Autodesk Fusion 360 part; units mm, degrees
sketch "Sketch1" plane through (0, 0, 0) normal (0, 0, 1) x (1, 0, 0) in component "test"
  line L0 (-10, 10) -> (5, 10)
  line L1 (5, 10) -> (5, 0)
  line L2 (5, 0) -> (-10, 0)
  line L3 (-10, 0) -> (-10, 10)
  line L4 (5, 0) -> (10, 0)
  line L5 (10, 0) -> (5, 2.5)
  dimension "d1" = 15
  dimension "d2" = 10
extrude "Extrude1" add sketch "Sketch1" along normal blind 0.5 in component "test"
sketch "Sketch2" plane through (0, 0, 0.5) normal (0, 0, 1) x (-1, 0, 0) in component "test"
  line L0 (10, 0) -> (-10, 0)
  line L1 (-5, -2.5) -> (-5, -10)
  line L2 (-5, -10) -> (10, -10)
  line L3 (10, -10) -> (10, 0)
  line L4 (10, -10) -> (9, -10)
  line L5 (9, -10) -> (9, 0)
  line L6 (9, 0) -> (10, 0)
  line L7 (10, 0) -> (10, -10)
  line L8 (-5, -10) -> (5, -10)
  line L9 (5, -10) -> (5, -8)
  line L10 (5, -8) -> (-5, -8)
  line L11 (-5, -8) -> (-5, -10)
  line L12 (-10, 0) -> (-5, -2.5)
extrude "Extrude2" add sketch "Sketch2" along normal blind 2 contours L0 L2 L3 L4 L5 L6 L7 | L1 L2 L8 L9 L10 L11 in component "test"
sketch "Sketch3" plane through (0, 0, 2.5) normal (0, 0, 1) x (-1, 0, 0) in component "test"
  line L0 (-5, -8) -> (-5, -10)
  line L1 (-5, -10) -> (5, -10)
  line L2 (5, -10) -> (5, -8)
  line L3 (5, -8) -> (-5, -8)
  line L4 (-5, -8) -> (4, -8)
  line L5 (4, -8) -> (4, -9)
  line L6 (4, -9) -> (-5, -9)
  line L7 (-5, -9) -> (-5, -8)
extrude "Extrude3" cut sketch "Sketch3" against normal blind 1.5 contours L0 L3 L4 L5 L6 L7 in component "test"
sketch "Sketch4" plane through (0, 0, 0.5) normal (0, 0, 1) x (-1, 0, 0) in component "test"
  line L0 (5, -8) -> (5, -10)
  line L1 (5, -10) -> (9, -10)
  line L2 (9, -10) -> (9, 0)
  line L3 (9, 0) -> (-10, 0)
  line L4 (-5, -2.5) -> (-5, -8)
  line L5 (-5, -8) -> (5, -8)
  line L6 (0, -7) -> (4, -7)
  line L7 (4, -7) -> (4, -2)
  line L8 (4, -2) -> (0, -2)
  line L9 (0, -2) -> (0, -7)
  circle A0 centre (6.5, -6.5) radius 1.5
  circle A1 centre (6.5, -2.5) radius 1
  line L10 (-10, 0) -> (-5, -2.5)
  dimension "d9" = 3
  dimension "d10" = 2
extrude "Extrude4" cut sketch "Sketch4" against normal through all contours L6 L7 L8 L9 | A0 | A1 in component "test"
sketch "Sketch5" plane through (0, 0, 2.5) normal (0, 0, 1) x (-1, 0, 0) in component "test"
  line L0 (10, 0) -> (9, 0)
  line L1 (9, 0) -> (9, -10)
  line L2 (9, -10) -> (10, -10)
  line L3 (10, -10) -> (10, 0)
  line L4 (10, -10) -> (2.5, -10)
  line L5 (2.5, -10) -> (2.5, -9)
  line L6 (2.5, -9) -> (10, -9)
  line L7 (10, -9) -> (10, -10)
extrude "Extrude5" add sketch "Sketch5" along normal blind 1 contours L1 L2 L3 L4 L6 L7 | L1 L4 L5 L6 in component "test"
chamfer "Chamfer1" distance 2.5 angle 45 1 edges at (-9.5, 0, 2.5) in component "test"
fillet "Fillet1" radius 2 1 edges at (5, 10, 1.25) in component "test"
fillet "Fillet2" radius 2 1 edges at (-4, 7, 0.25) in component "test"
sketch "Sketch6" plane through (0, 0, 0.5) normal (0, 0, 1) x (-1, 0, 0) in component "test"
  line L0 (9, -0.5) -> (-9, -0.5)
  line L1 (-9, -0.5) -> (-5, -2.5)
  line L2 (-5, -2.5) -> (-5, -8)
  line L3 (-5, -8) -> (5, -8)
  line L4 (5, -8) -> (5, -10)
  line L5 (5, -10) -> (9, -10)
  line L6 (9, -10) -> (9, -0.5)
  line L7 (0, -2) -> (4, -2)
  line L8 (4, -2) -> (4, -5)
  arc A0 (2, -7) -> (4, -5) centre (2, -5) ccw
  line L9 (2, -7) -> (0, -7)
  line L10 (0, -7) -> (0, -2)
  circle A1 centre (6.5, -6.5) radius 1.5
  circle A2 centre (6.5, -2.5) radius 1
  line L11 (5, -8.5) -> (9, -8.5)
  line L12 (9, -8.5) -> (9, -10)
  line L13 (9, -10) -> (5, -10)
  line L14 (5, -10) -> (5, -8.5)
extrude "Extrude6" cut sketch "Sketch6" against normal blind 0.3 contours L4 L5 L6 L11 L12 L13 L14 in component "test"
component "test" placed x (1, 0, 0) y (0, 1, 0) z (0, 0, 1) at (0, 0, 0)
Geometry: final body of the model. Coordinates: model frame, mm. A direction names the side the tool comes from. Round coordinates to 2 decimals unless told otherwise and drop trailing zeros. Order: outer loops, then holes, each group sorted by start corner. A loop starts at its lowest first (then second) coordinate and runs counter-clockwise, first axis right, second up.
Q1. Section C-C, the plane z = 2. Output: boundary loops of the cut face in (x, y).
Result sheet:
outline: (-10, 2) - (-9, 2) - (-9, 10) - (-10, 10) - close; (-5, 8) - (-4, 8) - (-4, 9) - (4.73, 9) arc R2 ccw to (3, 10) - (-5, 10) - close
Q2. Material intervals for probe 1 along Y at (x, z) = (-6.5, 0.25); probe 2 along Y at (x, z) = (-6.5, 0.35); probe 3 along Z at (x, y) = (0.75, 2.5), sorted ascending.
Result sheet:
probe 1: y = 0.25 to 1.5, 3.5 to 5, 8 to 8.5
probe 2: y = 0.35 to 1.5, 3.5 to 5, 8 to 8.5
probe 3: z = 0 to 0.5
Q3. Pin query (flat end, axial travel): pin 1 (0.6 mm diameter, centred on y = 6.5, z = 0, fed in from +X); pin 2 (0.5 mm diameter, centred on y = 8.5, z = 2, fed in from +X); pin 3 (1 mm diameter, centred on x = -3, y = 4, fed in from -Z); pin 4 (0.8 mm diameter, centred on x = 1, y = 9.5, fed in from +Z). Return the tip coordinate at first contact, or that it passes through.
Result sheet:
pin 1: stops at x = 5
pin 2: stops at x = -4
pin 3: passes through
pin 4: stops at z = 2.5
Q4. Access query for faces 1 (the face through (-7, 9.5, 2.5)), 2 (the face through (-4.5, 8.5, 2.5)), 3 (the face through (-2.5, 9.5, 3)), 4 (the face through (0.6, 8.5, 1)). Directions: +Z, -Z, +X, -X, +Y, -Y. A direction counts if a zero-diameter tool reaches every point of the face in a straight line with its end or side. Return the directions, or none.
Result sheet:
face 1: +Y, -Y
face 2: +Z, +X, -X, -Y
face 3: +Z, +X, +Y, -Y
face 4: +Z, +X, -Y
Q5. Section D-D, the plane y = 6.5. Output: boundary loops of the cut face in (x, z), and give its area (3 significant figures).
Result sheet:
outline: (-10, 0) - (-8, 0) - (-8, 0.5) - (-9, 0.5) - (-9, 2.5) - (-10, 2.5) - close; (-5, 0) - (-3.32, 0) - (-3.32, 0.5) - (-5, 0.5) - close; (0, 0) - (5, 0) - (5, 0.5) - (0, 0.5) - close
area: 6.34 mm2
Q6. Mould query, pull axis Y, two halves, no side actions, for faces 5 (the face through (-5.3, 7.4, 0.3)), 6 (the face through (-5.7, 3.1, 0.3)), 7 (the face through (-1.5, 0.3, 0.3)), 8 (the face through (-9.5, 5.7, 2.5)). Classes: released by +Y, released by -Y, zero draft, split by the parting line, or undercut.
Result sheet:
face 5: undercut
face 6: undercut
face 7: released by -Y
face 8: zero draft
Q7. Section B-B, the plane y = 3.75. Output: boundary loops of the cut face in (x, z).
Result sheet:
outline: (-10, 0) - (-4, 0) - (-4, 0.5) - (-9, 0.5) - (-9, 2.5) - (-10, 2.5) - close; (0, 0) - (5, 0) - (5, 0.5) - (0, 0.5) - close
Q8. Section A-A, the plane x = -6.5. Give the number of separate pieces and of enclosed holes in the cut face, and give its area (3 significant figures).
Result sheet:
separate pieces: 4
enclosed holes: 0
area: 2.93 mm2
